Work out the finished part from the listing and answer in its coordinate system (mm). Give positions to 0.01 mm unless a question says otherwise; leave off trailing zeros. Answer as a JSON object with one key per item and string values. Group by question number.
```python
from build123d import *

# Parameters (mm, degrees)
F4_R     = 2.6
F5_DEPTH = 12.901


with BuildPart() as f3:
    # F0 (on Front) → F3 section 0
    with BuildSketch(Plane.XZ):
        with BuildLine():
            Line((-27.112, 12.1), (-41.362, 12.1))
            Line((-41.362, 12.1), (-41.362, 11.3))
            Line((-41.362, 11.3), (-27.112, 11.3))
            ThreePointArc((-27.112, 11.3), (-26.404893, 11.007107), (-26.112, 10.3))
            ThreePointArc((-26.112, 10.3), (-22.860885, 2.451115), (-15.012, -0.8))
            Line((-15.012, -0.8), (15.012, -0.8))
            ThreePointArc((15.012, -0.8), (22.860885, 2.451115), (26.112, 10.3))
            ThreePointArc((26.112, 10.3), (26.404893, 11.007107), (27.112, 11.3))
            Line((27.112, 11.3), (41.362, 11.3))
            Line((41.362, 11.3), (41.362, 12.1))
            Line((41.362, 12.1), (27.112, 12.1))
            ThreePointArc((27.112, 12.1), (25.839208, 11.572792), (25.312, 10.3))
            ThreePointArc((25.312, 10.3), (22.2952, 3.0168), (15.012, 0))
            Line((15.012, 0), (-15.012, 0))
            ThreePointArc((-15.012, 0), (-22.2952, 3.0168), (-25.312, 10.3))
            ThreePointArc((-25.312, 10.3), (-25.839208, 11.572792), (-27.112, 12.1))
        make_face()
    # F2 (on offset) → F3 section 1
    with BuildSketch(Plane.XZ.offset(-80)):
        with BuildLine():
            Line((-28.387997, 12.1), (-42.637997, 12.1))
            Line((-42.637997, 12.1), (-42.637997, 11.3))
            Line((-42.637997, 11.3), (-28.387997, 11.3))
            ThreePointArc((-28.387997, 11.3), (-27.680891, 11.007107), (-27.387997, 10.3))
            ThreePointArc((-27.387997, 10.3), (-24.136883, 2.451115), (-16.287997, -0.8))
            Line((-16.287997, -0.8), (16.288003, -0.8))
            ThreePointArc((16.288003, -0.8), (24.136888, 2.451115), (27.388003, 10.3))
            ThreePointArc((27.388003, 10.3), (27.680896, 11.007107), (28.388003, 11.3))
            Line((28.388003, 11.3), (42.638003, 11.3))
            Line((42.638003, 11.3), (42.638003, 12.1))
            Line((42.638003, 12.1), (28.388003, 12.1))
            ThreePointArc((28.388003, 12.1), (27.11521, 11.572792), (26.588003, 10.3))
            ThreePointArc((26.588003, 10.3), (23.571203, 3.0168), (16.288003, 0))
            Line((16.288003, 0), (-16.288003, 0))
            ThreePointArc((-16.288003, 0), (-23.571199, 3.016802), (-26.587997, 10.3))
            ThreePointArc((-26.587997, 10.3), (-27.115205, 11.572792), (-28.387997, 12.1))
        make_face()
    loft()

    # F4 (on face) → F5 (cut, through all)
    with BuildSketch(Plane.XY.offset(12.1)):
        with Locations((-35.055441, 71.748368)):
            Circle(F4_R)
        with Locations((-34.768377, 53.750657)):
            Circle(F4_R)
        with Locations((-34.337781, 26.754091)):
            Circle(F4_R)
        with Locations((-34.050717, 8.75638)):
            Circle(F4_R)
        with BuildLine():
            ThreePointArc((36.650386, 8.714916), (36.650634, 8.735647), (36.650717, 8.75638))
            ThreePointArc((36.650717, 8.75638), (31.4508, 8.777113), (36.650386, 8.714916))
        make_face()
        with BuildLine():
            ThreePointArc((36.93745, 26.712626), (36.937698, 26.733358), (36.937781, 26.754091))
            ThreePointArc((36.937781, 26.754091), (31.737864, 26.774824), (36.93745, 26.712626))
        make_face()
        with BuildLine():
            ThreePointArc((37.368047, 53.709193), (37.368295, 53.729924), (37.368377, 53.750657))
            ThreePointArc((37.368377, 53.750657), (32.16846, 53.77139), (37.368047, 53.709193))
        make_face()
        with BuildLine():
            ThreePointArc((37.655111, 71.706903), (37.655359, 71.727635), (37.655441, 71.748368))
            ThreePointArc((37.655441, 71.748368), (32.455524, 71.769101), (37.655111, 71.706903))
        make_face()
    extrude(amount=-F5_DEPTH, mode=Mode.SUBTRACT)


solid = f3.part
```
Item 1: Given pin 1 Ø1 at (y, z) = (27.5, 6.5) entering from +X; pin 2 Ø4.5 at (x, y) = (-34.05, 8.76) entering from +Z; pin 3 Ø4 at (x, y) = (-8.5, 38) entering from +Z; pin 4 Ø4 at (y, z) = (70.5, 10.5) entering from +X, each flat-ended and moving along its own axis, determine where each tip first touches the part or whether it passes through.
Item 2: For a pull along X with two mould halves and no side action, classify faces 1 (the cylindrical face through (-35.97, 10.51, 11.71)), 2 (the flat face through (0.2, 80, -0.6)) as pulls with the +X half, pulls with the -X half, needs draft (parallel to the pull), parting line crosses it, or undercut.
Item 3: Find the intervals of material crossed by probe 1 along X at (y, z) = (5.5, 9); probe 2 along Z at (x, y) = (15, 9.5); probe 3 along Z at (x, y) = (39, 39.5), in increasing order. Write a range as [from, to].
The answers:
{
 "1": {"pin 1": "stops at x = 26.05", "pin 2": "passes through", "pin 3": "stops at z = 0", "pin 4": "stops at x = 42.52"},
 "2": {"face 1": "undercut", "face 2": "needs draft"},
 "3": {"probe 1": "x = [-26.12, -25.32], [25.32, 26.12]", "probe 2": "z = [-0.8, 0]", "probe 3": "z = [11.3, 12.1]"}
}
